CAD build for the part. Positions are in the model's coordinates, mm. A direction names the side the tool comes from. Coordinates: 2 decimals unless noted, no trailing zeros. Loops run counter-clockwise (first coordinate to the right, second up) from the corner with the lowest first, then second, coordinate; pieces in that order, holes last. Notation, with made-up numbers: (5.25, 34) -> (11.25, 34) arc R14 cw to (11.25, 41) -> close; hole circle Ø1 at (42.5, -13). An arc over 180 degrees is marked (long way). Return JSON: item names as keys, results as strings. Group by question number.
(1) Saw through at C-C on y = 0.8. Write the cut outline in (x, z), then the cut area to 3 significant figures.
(2) Mould opens along X. For faces 1 (the face through (-36.95, 1.01, 1.94)), 2 (the face through (-6, 0, 37)), 3 (the face through (-40.943, 1.479, 2.155)) say: pulls with the +X half, pulls with the -X half, needs draft (parallel to the pull), parting line crosses it, or undercut.
(3) Saw through at B-B on x = 0. Write the cut outline in (y, z).
(4) Tool access for faces 4 (the face through (-8.9, 3, -39.3)), 5 (the face through (39, 1, 0)), 6 (the face through (-11.7, 2, -35.4)): list every direction of +Z, -Z, +X, -X, +Y, -Y with a clear straight run to the whole face (end or side of a thin tool).
(5) Probe L1, parallel to X at y = 0.9, z = -1; L2, parallel to Z at x = 0, y = 2.3; L3, parallel to Z at x = 0, y = 1.15. List the from-to ranges inside material, lowest first.
(6) Saw through at A-A on z = 22. Write the cut outline in (x, y), then the cut area to 3 significant figures.
```python
from build123d import *

# Parameters (mm, degrees)
REVOLVE_1_ANGLE = 359


with BuildPart() as part:
    # 草图1 → 旋转1 (revolve)
    with BuildSketch(Plane.XY):
        Polygon((40, 3), (41, 3), (41, 0), (37, 0), (37, 2), (40, 2), align=None)
    revolve(axis=Axis((0, 10, 0), (0, -1, 0)), revolution_arc=REVOLVE_1_ANGLE)


solid = part.part
```
Geometry results:
{
 "1": {"outline": "(36.99, -0.65) arc R37 cw (long way) to (37, 0) -> (41, 0) arc R41 ccw (long way) to (40.99, -0.72) -> close", "area": "977 mm²"},
 "2": {"face 1": "undercut", "face 2": "needs draft", "face 3": "parting line crosses it"},
 "3": {"outline": "(0, -41) -> (3, -41) -> (3, -40) -> (2, -40) -> (2, -37) -> (0, -37) -> close; (0, 37) -> (2, 37) -> (2, 40) -> (3, 40) -> (3, 41) -> (0, 41) -> close"},
 "4": {"face 4": "+Z, -Z, +X, -X, +Y", "face 5": "+X, +Y, -Y", "face 6": "+Y"},
 "5": {"L1": "-40.99 to -36.99, 36.99 to 40.99", "L2": "-41 to -40, 40 to 41", "L3": "-41 to -37, 37 to 41"},
 "6": {"outline": "(-34.6, 0) -> (-29.75, 0) -> (-29.75, 2) -> (-33.41, 2) -> (-33.41, 3) -> (-34.6, 3) -> close; (29.75, 0) -> (34.6, 0) -> (34.6, 3) -> (33.41, 3) -> (33.41, 2) -> (29.75, 2) -> close", "area": "21.8 mm²"}
}
